Check sheet for the modelled part. Datum: model origin and axes. Units: mm. Give positions to 0.01 mm unless a question says otherwise; leave off trailing zeros. Order: outer loops, then holes, each group sorted by start corner. A loop starts at its lowest first (then second) coordinate and runs counter-clockwise, first axis right, second up. Notation, with made-up numbers: M 77,78 L 88,78 A23 cw 88,110 Z; hole C 47,-3.5 d7. An arc over 180 degrees is marked long. One line per question, with ' | ' between items. Start each with the question number.
```python
from build123d import *

# Parameters (mm, degrees)
BOSS_EXTRUDE1_DEPTH = 30
SKETCH2_R           = 4.2
CUT_EXTRUDE1_DEPTH  = 31


with BuildPart() as part:
    # Sketch1 → Boss-Extrude1 (new body)
    with BuildSketch(Plane.XY):
        Polygon((0, 9.814954576), (-8.5, 4.907477288), (-8.5, -4.907477288), (0, -9.814954576), (8.5, -4.907477288), (8.5, 4.907477288), align=None)
    extrude(amount=BOSS_EXTRUDE1_DEPTH)

    # Sketch2 → Cut-Extrude1 (cut, through all)
    with BuildSketch(Plane.XY.offset(30)):
        Circle(SKETCH2_R)
    extrude(amount=-CUT_EXTRUDE1_DEPTH, mode=Mode.SUBTRACT)

    # Sketch3 → Cut-Revolve1 (revolve, cut)
    with BuildSketch(Plane(origin=(0, 0, 0), x_dir=(0, 0, -1), z_dir=(1, 0, 0))):
        Polygon((-28.661748937, 9.814954576), (-30, 7.798581685), (-30, 9.814954576), align=None)
        Polygon((0, 7.798581685), (0, 9.814954576), (-1.338251063, 9.814954576), align=None)
    revolve(axis=Axis((0, 0, -5.872116431), (0, 0, 1)), mode=Mode.SUBTRACT)


solid = part.part
```
Item 1: Section check B-B, the plane y = 0. Record the cut outline in (x, z), then the cut area to 3 significant figures.
Item 2: Scan lines: probe 1 along Y at (x, z) = (-2.75, 11.25); probe 2 along X at (y, z) = (-2.75, 25.75); probe 3 along X at (y, z) = (-3.25, 28.25). Record each from-to range of solid material in increasing order. Write a range as [from, to].
Item 3: Draft check along X on faces 1 (the face through (4.006, 1.262, 15.21)), 2 (the face through (4.191, -7.396, 14.797)), 3 (the face through (-4.309, -7.327, 14.797)). Enter one of: released by +X, released by -X, zero draft, split by the parting line, or undercut.
Item 4: Section check A-A, the plane z = 9.75. Record the cut outline in (x, y), then the cut area to 3 significant figures.
Item 5: Go/stop test with flat-tipped pins: P1, Ø4, axis at x = 4, z = 19.5, coming from the -Y side; P2, Ø5, axis at x = 3.5, z = 12.5, coming from the -Y side; P3, Ø1.5, axis at x = -5, z = 17.5, coming from the +Y side. Record where each tip stops, or that it passes through.
Reported:
1) outline: M -8.5,0.47 L -7.8,0 L -4.2,0 L -4.2,30 L -7.8,30 L -8.5,29.53 Z; M 4.2,0 L 7.8,0 L 8.5,0.47 L 8.5,29.53 L 7.8,30 L 4.2,30 Z | area: 257 mm^2
2) probe 1: y = [-8.23, -3.17], [3.17, 8.23] | probe 2: x = [-8.5, -3.17], [3.17, 8.5] | probe 3: x = [-8.5, -2.66], [2.66, 8.5]
3) face 1: undercut | face 2: released by +X | face 3: released by -X
4) outline: M -8.5,-4.91 L 0,-9.81 L 8.5,-4.91 L 8.5,4.91 L 0,9.81 L -8.5,4.91 Z; hole C 0,0 d8.4 | area: 195 mm^2
5) P1: stops at y = -8.66 | P2: stops at y = -9.24 | P3: stops at y = 7.36
